```python
from build123d import *

# Parameters (mm, degrees)
SKETCH1_W            = 60
SKETCH1_H            = 45
BOSS_EXTRUDE1_DEPTH  = 3
SKETCH2_R            = 2
CUT_EXTRUDE1_DEPTH   = 5
CUT_EXTRUDE5_DEPTH   = 2
CUT_EXTRUDE4_DEPTH   = 5
CHAMFER2_SIZE        = 1
FILLET1_R            = 4
FILLET1_OF_MIRROR4_R = 4
CHAMFER1_SIZE        = 1


with BuildPart() as part:
    # Sketch1 → Boss-Extrude1 (new body)
    with BuildSketch(Plane.XY):
        Rectangle(SKETCH1_W, SKETCH1_H)
    extrude(amount=BOSS_EXTRUDE1_DEPTH)

    # Sketch2 → Cut-Extrude1 (cut)
    with BuildSketch(Plane(origin=(0, 0, 0), x_dir=(-1, 0, 0), z_dir=(0, 0, -1))):
        with Locations((19.5, 0)):
            Circle(SKETCH2_R)
        with Locations((25.5, 6)):
            Circle(SKETCH2_R)
        with Locations((25.5, -6)):
            Circle(SKETCH2_R)
        with Locations((19.5, -12)):
            Circle(SKETCH2_R)
        with Locations((19.5, 12)):
            Circle(SKETCH2_R)
    cut_extrude1 = extrude(amount=-CUT_EXTRUDE1_DEPTH, mode=Mode.SUBTRACT)

    # Sketch8 → Cut-Extrude5 (cut)
    with BuildSketch(Plane.XY.offset(3)):
        Polygon((-14, 4), (-14, -4), (-25, -12), (-30, -12), (-30, 12), (-25, 12), align=None)
    cut_extrude5 = extrude(amount=-CUT_EXTRUDE5_DEPTH, mode=Mode.SUBTRACT)

    # Sketch7 → Cut-Extrude4 (cut)
    with BuildSketch(Plane.XY.offset(3)):
        with BuildLine():
            Line((-11, -18.5), (9, -18.5))
            Line((9, -18.5), (9, -11.5))
            Line((9, -11.5), (-11, -11.5))
            ThreePointArc((-11, -11.5), (-14.5, -15), (-11, -18.5))
        make_face()
        with BuildLine():
            Line((-11, 11.5), (9, 11.5))
            Line((9, 11.5), (9, 18.5))
            Line((9, 18.5), (-11, 18.5))
            ThreePointArc((-11, 18.5), (-14.5, 15), (-11, 11.5))
        make_face()
    cut_extrude4 = extrude(amount=-CUT_EXTRUDE4_DEPTH, mode=Mode.SUBTRACT)

    # Chamfer2
    chamfer2_edges = [part.edges().sort_by_distance(p)[0] for p in [
        (0, -22.5, 3),
        (0, 22.5, 3),
    ]]
    chamfer(chamfer2_edges, length=CHAMFER2_SIZE)

    # Fillet1
    fillet1_edges = [part.edges().sort_by_distance(p)[0] for p in [
        (-25, 12, 2),
        (-14, 4, 2),
        (-14, -4, 2),
        (-25, -12, 2),
    ]]
    fillet(fillet1_edges, radius=FILLET1_R)

    # Mirror4: Cut-Extrude1, Cut-Extrude5, Cut-Extrude4 across plane
    add(cut_extrude1.mirror(Plane(origin=(0, 0, 0), x_dir=(0, 0, 1), z_dir=(1, 0, 0))), mode=Mode.SUBTRACT)
    add(cut_extrude5.mirror(Plane(origin=(0, 0, 0), x_dir=(0, 0, 1), z_dir=(1, 0, 0))), mode=Mode.SUBTRACT)
    add(cut_extrude4.mirror(Plane(origin=(0, 0, 0), x_dir=(0, 0, 1), z_dir=(1, 0, 0))), mode=Mode.SUBTRACT)

    # Fillet1 of Mirror4
    fillet1_of_mirror4_edges = [part.edges().sort_by_distance(p)[0] for p in [
        (25, 12, 2),
        (14, 4, 2),
        (14, -4, 2),
        (25, -12, 2),
    ]]
    fillet(fillet1_of_mirror4_edges, radius=FILLET1_OF_MIRROR4_R)

    # Chamfer1
    chamfer1_edges = [part.edges().sort_by_distance(p)[0] for p in [
        (14.5, -15, 3),
        (14.5, 15, 3),
        (-14.5, -15, 3),
        (0, -18.5, 3),
        (0, -11.5, 3),
        (0, 18.5, 3),
        (-14.5, 15, 3),
        (0, 11.5, 3),
    ]]
    chamfer(chamfer1_edges, length=CHAMFER1_SIZE)


solid = part.part
```
For this review, take the finished solid that the model builds, in its own axes (mm). A direction names the side the tool comes from. Round coordinates to 2 decimals unless told otherwise and drop trailing zeros. Loops run counter-clockwise (first coordinate to the right, second up) from the corner with the lowest first, then second, coordinate; pieces in that order, holes last.
Q1. Add section B-B on y = -15. Write out the cut boundary in (x, z), plus the area to 3 significant figures.
Result sheet:
outline: (-30, 0) - (-14.5, 0) - (-14.5, 2) - (-15.5, 3) - (-30, 3) - close; (14.5, 0) - (30, 0) - (30, 3) - (15.5, 3) - (14.5, 2) - close
area: 92.0 mm2
Q2. Insertion check: pin 1 Ø6.5 at (x, y) = (25.5, -6) entering from +Z; pin 2 Ø1.6 at (y, z) = (-0.5, 2.5) entering from +X; pin 3 Ø3.5 at (x, y) = (19.5, 0) entering from +Z. Each pin has a flat end and moves straight along its axis. Give the tip position at first contact, or say it passes through.
Result sheet:
pin 1: stops at z = 1
pin 2: stops at x = 14
pin 3: passes through
Q3. Add section D-D on y = 6. Write out the cut boundary in (x, z), plus the area to 3 significant figures.
Result sheet:
outline: (-30, 0) - (-27.5, 0) - (-27.5, 1) - (-30, 1) - close; (-23.5, 0) - (23.5, 0) - (23.5, 1) - (16.75, 1) - (16.75, 3) - (-16.75, 3) - (-16.75, 1) - (-23.5, 1) - close; (27.5, 0) - (30, 0) - (30, 1) - (27.5, 1) - close
area: 119 mm2
Q4. Mouldability with a two-part tool opening along Y and no side actions: class faces 1 (the face through (-30, -0.3, 0.8)), 2 (the face through (-18.026, -10.648, 1.479)) as +Y half, -Y half, draft (parallel to the pull), parting line (faces both ways), or undercut.
Result sheet:
face 1: draft
face 2: undercut
Q5. Machinability: for faces 3 (the face through (0, -11.5, 1)), 4 (the face through (14, 0, 2)), 5 (the face through (-25.08, -11.81, 1.99)), 6 (the face through (-14.7, -15.1, 2.2)), which of the approach directions +Z, -Z, +X, -X, +Y, -Y give a long, thin tool a straight path to every point of the face, cutting with its end or side? Answer none if there is none.
Result sheet:
face 3: +Z, -Z
face 4: +Z, +X
face 5: +Z, -X
face 6: +Z
Q6. To check wall thickness, follow line 1 along Y through (x, z) = (7, 0.2); line 2 along Y through (x, z) = (-19.5, 0.3); line 3 along Y through (x, z) = (-19.5, 1.9). State the ranges of each line that lie inside material, in increasing order.
Result sheet:
line 1: y = -22.5 to -18.5, -11.5 to 11.5, 18.5 to 22.5
line 2: y = -22.5 to -14, -10 to -2, 2 to 10, 14 to 22.5
line 3: y = -22.5 to -14, -10 to -8, 8 to 10, 14 to 22.5
Q7. Add section C-C on z = 0.5. Give the number of separate pieces and of enclosed holes in the cut face, plus the area to 3 significant figures.
Result sheet:
separate pieces: 1
enclosed holes: 12
area: 2,190 mm2
Q8. Add section A-A on x = -4. Write out the cut boundary in (y, z), plus the area to 3 significant figures.
Result sheet:
outline: (-22.5, 0) - (-18.5, 0) - (-18.5, 2) - (-19.5, 3) - (-21.5, 3) - (-22.5, 2) - close; (-11.5, 0) - (11.5, 0) - (11.5, 2) - (10.5, 3) - (-10.5, 3) - (-11.5, 2) - close; (18.5, 0) - (22.5, 0) - (22.5, 2) - (21.5, 3) - (19.5, 3) - (18.5, 2) - close
area: 90.0 mm2
